For this review, take the finished solid that the model builds, in its own axes (mm). Coordinates: 2 decimals unless noted, no trailing zeros. Loops run counter-clockwise (first coordinate to the right, second up) from the corner with the lowest first, then second, coordinate; pieces in that order, holes last. Notation, with made-up numbers: (74.5, 19.5) - (86.5, 19.5) arc R23 cw to (86.5, 45.5) - close; hole circle Ø9 at (-13.5, -5.5). An arc over 180 degrees is marked (long way). Answer as a JSON object with one key per item and string values. Group by question number.
Item 1: We need section A-A (y = 0). Give the boundary of the cut face in (x, z), then the cut area to 3 significant figures.
Item 2: Clearance check with flat-ended pins moving along their axes: pin 1 (1 mm diameter, centred on x = 2, y = -29.5, fed in from -Z); pin 2 (1 mm diameter, centred on x = 2.5, z = -27.5, fed in from -Y); pin 3 (1.5 mm diameter, centred on x = 2.5, y = -28.5, fed in from +Z). State where each tip first meets the part, or that it passes through.
Item 3: To check wall thickness, follow line 1 (Z direction, x = 1.25, y = 1.5); line 2 (Y direction, x = 1.1, z = -43.5); line 3 (Y direction, x = 1.9, z = -3). State the ranges of each line that lie inside material, in increasing order.
Item 4: We need section C-C (y = -50). Give the boundary of the cut face in (x, z), then the cut area to 3 significant figures.
Autodesk Inventor part; units mm, degrees
ref_plane "YZ Plane" through (0, 0, 0) normal (1, 0, 0) x (0, 1, 0)
ref_plane "XZ Plane" through (0, 0, 0) normal (0, 1, 0) x (-1, 0, 0)
ref_plane "XY Plane" through (0, 0, 0) normal (0, 0, 1) x (1, 0, 0)
sketch "Sketch1" plane through (0, 0, 0) normal (1, 0, 0) x (0, 1, 0)
  circle A0 centre (0, 0) radius 62.5
  dimension "d0" = 125
extrude "Extrusion1" add sketch "Sketch1" along normal blind 5
sketch "Sketch2" plane through (5, 0, 0) normal (1, 0, 0) x (0, 0, -1)
  circle A0 centre (0, 50) radius 3.5
  circle A1 centre (-50, 0) radius 3.5
  circle A2 centre (0, -50) radius 3.5
  circle A3 centre (50, 0) radius 3.5
  circle A4 centre (-43.3013, -25) radius 3.5
  circle A5 centre (43.3013, -25) radius 3.5
  circle A6 centre (0, 0) radius 3.5
  dimension "d3" = 7
  dimension "d4" = 0
  dimension "d5" = 50
  dimension "d8" = 360
  dimension "d12" = 360
  dimension "d16" = 7
extrude "Extrusion2" cut sketch "Sketch2" against normal through all
properties part number "Base"
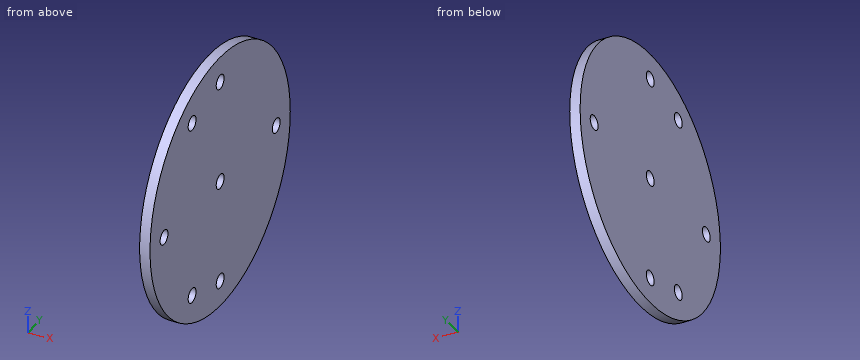
Check sheet entries:
{
 "1": {"outline": "(0, -62.5) - (5, -62.5) - (5, -53.5) - (0, -53.5) - close; (0, -46.5) - (5, -46.5) - (5, -3.5) - (0, -3.5) - close; (0, 3.5) - (5, 3.5) - (5, 46.5) - (0, 46.5) - close; (0, 53.5) - (5, 53.5) - (5, 62.5) - (0, 62.5) - close", "area": "520 mm2"},
 "2": {"pin 1": "stops at z = -55.36", "pin 2": "stops at y = -56.37", "pin 3": "stops at z = 56"},
 "3": {"line 1": "z = -62.48 to -53.16, -46.84 to -3.16, 3.16 to 46.84, 53.16 to 62.48", "line 2": "y = -44.88 to -28.49, -21.51 to 44.88", "line 3": "y = -62.43 to -51.8, -48.2 to -1.8, 1.8 to 48.2, 51.8 to 62.43"},
 "4": {"outline": "(0, -37.5) - (5, -37.5) - (5, -3.5) - (0, -3.5) - close; (0, 3.5) - (5, 3.5) - (5, 37.5) - (0, 37.5) - close", "area": "340 mm2"}
}
